The drawing under review shows one solid part. Ordinate dimensions are in mm from its lowest x, y, z. Give positions to 0.01 mm unless a question says otherwise; leave off trailing zeros. Loops run counter-clockwise (first coordinate to the right, second up) from the corner with the lowest first, then second, coordinate; pieces in that order, holes last.
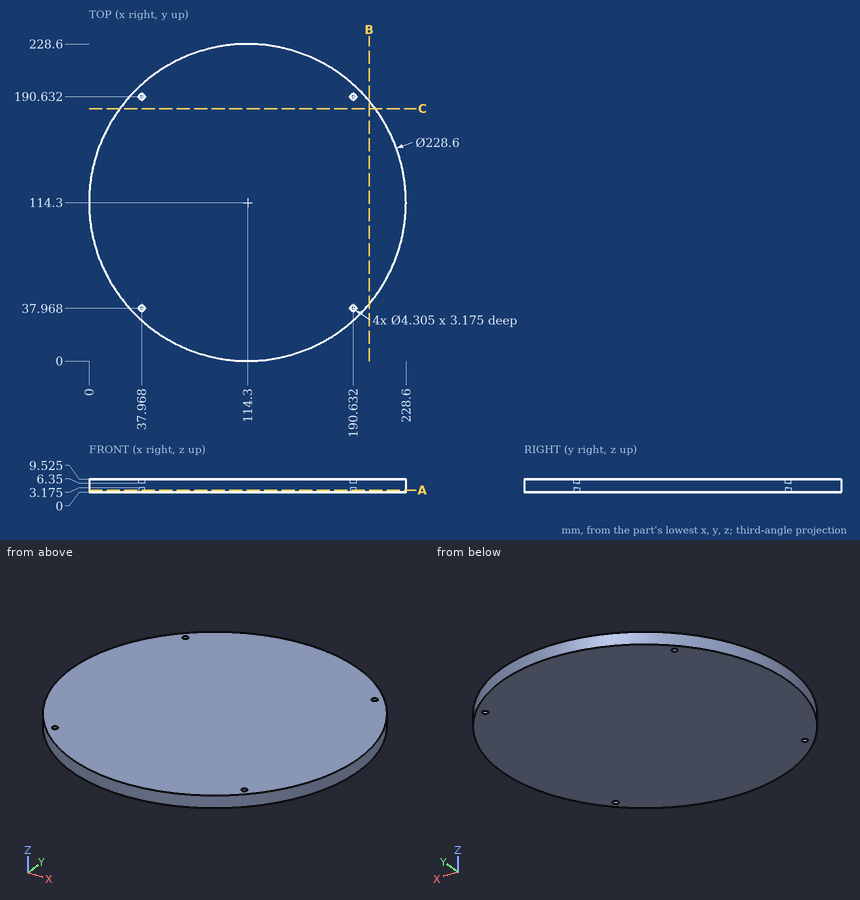
Item 1: For L1, parallel to X at y = 111, z = 3.75; L2, parallel to X at y = 143.5, z = 3.5; L3, parallel to Y at x = 29, z = 8, list the stretches that pass through material, from the lowest coordinate up.
Answer:
L1: x = 0.05 to 228.55
L2: x = 3.79 to 224.81
L3: y = 38.22 to 190.38
Item 2: Take a section at B-B on x = 202. Give the boundary of the cut face in (y, z) (1 decimal), and give its area (3 significant figures).
Answer:
outline: (41, 0) - (187.6, 0) - (187.6, 9.5) - (41, 9.5) - close
area: 1,400 mm2
Item 3: Take a section at A-A on z = 1.5. Give the boundary of the cut face in (x, y) (1 decimal), and give its area (3 significant figures).
Answer:
outline: circle Ø228.6 at (114.3, 114.3); hole circle Ø4.3 at (38, 38); hole circle Ø4.3 at (38, 190.6); hole circle Ø4.3 at (190.6, 38); hole circle Ø4.3 at (190.6, 190.6)
area: 41,000 mm2
Item 4: Take a section at C-C on y = 182. Give the boundary of the cut face in (x, z) (1 decimal).
Answer:
outline: (22.2, 0) - (206.4, 0) - (206.4, 9.5) - (22.2, 9.5) - close
Item 5: Clearance check with flat-ended pins moving along their axes: pin 1 Ø2 at (x, y) = (191, 190) entering from +Z; pin 2 Ø1 at (x, y) = (138, 183) entering from -Z; pin 3 Ø1.5 at (y, z) = (53, 7) entering from +X (1 decimal); pin 4 Ø2 at (x, y) = (191, 191) entering from -Z (3 decimals). State where each tip first meets the part, or that it passes through.
Answer:
pin 1: stops at z = 6.35
pin 2: stops at z = 0
pin 3: stops at x = 211.2
pin 4: stops at z = 3.175
